Solid Edge part; units mm, degrees
sketch "Sketch1" plane through (0, 0, 0) normal (0, 0, 1) x (1, 0, 0)
  line L0 (63, 7) -> (0, 15)
  arc A0 (0, 15) -> (0, -15) centre (-1.9048, 0) ccw
  line L1 (63, -7) -> (0, -15)
  arc A1 (63, 7) -> (63, -7) centre (62.1111, 0) cw
extrude "Protrusion1" add sketch "Sketch1" along normal blind 10
sketch "Sketch2" plane through (26.0711, 0, 0) normal (0, 0, -1) x (-0.992, -0.126, 0)
  circle A0 centre (25.8634, 3.2842) radius 14
extrude "ExtrudedProtrusion_3" add sketch "Sketch2" along normal blind 2
sketch "Sketch3" plane through (26.0711, 0, -2) normal (0, 0, -1) x (-1, 0, 0)
  circle A0 centre (26.0711, 0) radius 5
extrude "ExtrudedProtrusion_2" add sketch "Sketch3" along normal blind 42
sketch "Sketch4" plane through (0, 0, 0) normal (1, 0, 0) x (0, 1, 0)
  circle A0 centre (0, -38) radius 1
extrude "Cutout1" cut sketch "Sketch4" along normal mid plane 36.7222
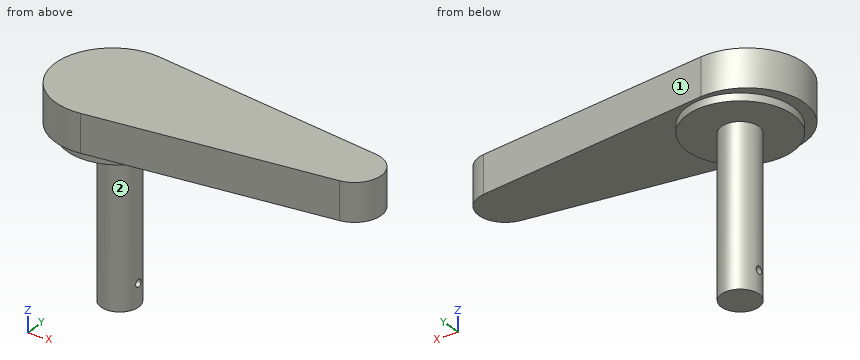
Model file for the job. Use its own axes, mm. Face numbers are marked on the shaded views. A direction names the side the tool comes from. Coordinates: 2 decimals unless noted, no trailing zeros. Loops run counter-clockwise (first coordinate to the right, second up) from the corner with the lowest first, then second, coordinate; pieces in that order, holes last. Notation, with made-up numbers: (0.5, 69.5) - (53.5, 69.5) arc R24 cw to (53.5, 90.5) - close; hole circle Ø3 at (4, 62.5). An arc over 180 degrees is marked (long way). Write item = value, one per line. Start each with the question number.
Item 1: Wall check: probe 1 along Z at (x, y) = (-1, 0); probe 2 along Z at (x, y) = (31.5, -5); probe 3 along Y at (x, z) = (-2, -38). Give the ranges that are in metal, low to high. Write a range as [from, to].
Item 2: Saw through at B-B, the plane z = -38. List the corners of the cut face in (x, y), then the cut area to 3 significant figures.
Item 3: 3-axis set-ups, long thin cutter, end or side, ignore diameter. For the marked faces 1 and 2: which of +Z, -Z, +X, -X, +Y, -Y reach the whole face in a straight line?
Item 4: Saw through at C-C, the plane x = 3. List the corners of the cut face in (y, z), then the cut area to 3 significant figures.
Item 5: Saw through at A-A, the plane y = 0. List the corners of the cut face in (x, z).
Item 6: Drop flat-ended pins along their axis: pin 1 Ø1.5 at (x, y) = (5, -5) entering from -Z; pin 2 Ø2.5 at (y, z) = (0, -38) entering from +X; pin 3 Ø8 at (x, y) = (26.5, 9.5) entering from -Z. Give the stop position or say it passes through.
Item 7: Saw through at D-D, the plane y = -10. List the corners of the cut face in (x, z) (3 decimals), then the cut area to 3 significant figures.
Answers:
q1.probe_1 = [-44, -39], [-37, 10]
q1.probe_2 = [0, 10]
q1.probe_3 = [-4.58, -1], [1, 4.58]
q2.outline = (-4.9, -1) arc R5 ccw to (4.9, -1) - close; (-4.9, 1) - (4.9, 1) arc R5 ccw to start
q2.area = 58.7 mm2
q3.face_1 = +Z, -Z, +X, +Y
q3.face_2 = -Z
q4.outline = (-14.62, 0) - (-13.68, 0) - (-13.68, -2) - (-4, -2) - (-4, -44) - (4, -44) - (4, -2) - (13.67, -2) - (13.67, 0) - (14.62, 0) - (14.62, 10) - (-14.62, 10) - close; hole circle Ø2 at (0, -38)
q4.area = 680 mm2
q5.outline = (-17.03, 0) - (-14, 0) - (-14, -2) - (-5, -2) - (-5, -37) - (5, -37) - (5, -2) - (14, -2) - (14, 0) - (69.17, 0) - (69.17, 10) - (-17.03, 10) - close; (-5, -44) - (5, -44) - (5, -39) - (-5, -39) - close
q6.pin_1 = -2
q6.pin_2 = 5
q6.pin_3 = 0
q7.outline = (-13.246, 0) - (-9.799, 0) - (-9.799, -2) - (9.799, -2) - (9.799, 0) - (39.375, 0) - (39.375, 10) - (-13.246, 10) - close
q7.area = 565 mm2
